Design review of the part built by this model. Coordinates are the model's own, in mm. Face numbers are marked on the shaded views. Coordinates: 2 decimals unless noted, no trailing zeros. Loops run counter-clockwise (first coordinate to the right, second up) from the corner with the lowest first, then second, coordinate; pieces in that order, holes last. Notation, with made-up numbers: M 25,-24.75 L 30,-24.75 A17 ccw 30,-3.75 Z; hole C 36.5,-34 d2. An arc over 180 degrees is marked long. One line per item, written item: value.
```python
from build123d import *

# Parameters (mm, degrees)
F0_W      = 67
F0_H      = 50
F1_DEPTH  = 70
F3_DEPTH  = 1.5
F4_W      = 29
F4_H      = 3.3
F5_DEPTH  = 67.001
F6_R      = 3.15
F7_DEPTH  = 9.2
F9_R      = 20
F10_DEPTH = 1.5
F12_R     = 20
F13_DEPTH = 1.5


with BuildPart() as f1:
    # F0 (on Top) → F1 (new body)
    with BuildSketch(Plane.XY):
        with Locations((33.5, 25)):
            Rectangle(F0_W, F0_H)
    extrude(amount=F1_DEPTH)

    # F2 (on face) → F3 (cut)
    with BuildSketch(Plane.XZ):
        Polygon((8.3138438763, 70), (0, 70), (0, 65.2), (28.9057142857, 35), (0, 4.8), (0, 0), (8.3138438763, 0), (33.5, 26.3138944576), (58.6861561237, 0), (67, 0), (67, 4.8), (38.0942857143, 35), (67, 65.2), (67, 70), (58.6861561237, 70), (33.5, 43.6861055424), align=None)
    extrude(amount=-F3_DEPTH, mode=Mode.SUBTRACT)

    # F4 (on face) → F5 (cut, through all)
    with BuildSketch(Plane.YZ.offset(67)):
        with BuildLine():
            Line((50, 36.5), (43.4544826719, 36.5))
            ThreePointArc((43.4544826719, 36.5), (8, 27), (43.4544826719, 17.5))
            Line((43.4544826719, 17.5), (50, 17.5))
            Line((50, 17.5), (50, 36.5))
        make_face()
        with Locations((35.5, 59.15)):
            Rectangle(F4_W, F4_H)
    extrude(amount=-F5_DEPTH, mode=Mode.SUBTRACT)

    # F6 (on face) → F7 (cut, through all)
    with BuildSketch(Plane.XY.offset(70)):
        with Locations((33.5, 41.7)):
            Circle(F6_R)
    extrude(amount=-F7_DEPTH, mode=Mode.SUBTRACT)

    # F9 (on offset) → F10 (cut)
    with BuildSketch(Plane.YZ.offset(54.5)):
        with Locations((27, 27)):
            Circle(F9_R)
    extrude(amount=F10_DEPTH, mode=Mode.SUBTRACT)

    # F12 (on offset) → F13 (cut)
    with BuildSketch(Plane(origin=(12.5, 0, 0), x_dir=(0, -1, 0), z_dir=(-1, 0, 0))):
        with Locations((-27, 27)):
            Circle(F12_R)
    extrude(amount=F13_DEPTH, mode=Mode.SUBTRACT)


solid = f1.part
```
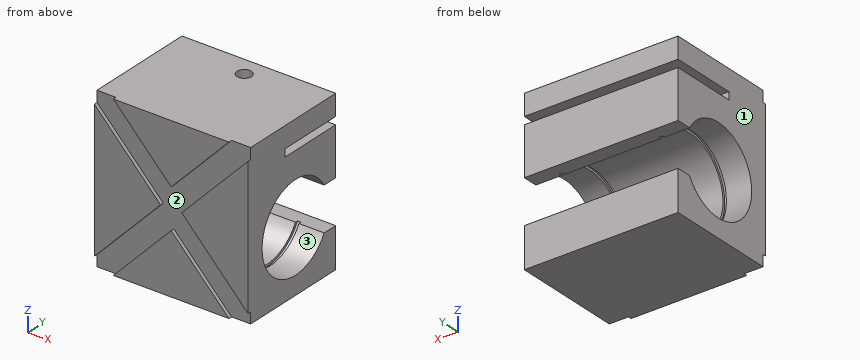
(1) To check wall thickness, follow line 1 along X through (y, z) = (9, 20.5); line 2 along Z through (x, y) = (61, 27); line 3 along Z through (x, y) = (55, 27). State the ranges of each line that lie inside material, in increasing order. Write a range as [from, to].
Reply:
line 1: x = [0, 11], [12.5, 54.5], [56, 67]
line 2: z = [0, 8], [46, 57.5], [60.8, 70]
line 3: z = [0, 7], [47, 57.5], [60.8, 70]
(2) Insertion check: pin 1 (4 mm diameter, centred on x = 33.5, y = 41.7, fed in from +Z); pin 2 (2.5 mm diameter, centred on x = 49.5, z = 59.5, fed in from +Y). Each pin has a flat end and moves straight along its axis. Give the tip position at first contact, or say it passes through.
Reply:
pin 1: stops at z = 57.5
pin 2: stops at y = 21
(3) We need section A-A on y = 27. State the section outline as (x, z) points.
Reply:
outline: M 0,0 L 67,0 L 67,8 L 56,8 L 56,7 L 54.5,7 L 54.5,8 L 12.5,8 L 12.5,7 L 11,7 L 11,8 L 0,8 Z; M 0,46 L 11,46 L 11,47 L 12.5,47 L 12.5,46 L 54.5,46 L 54.5,47 L 56,47 L 56,46 L 67,46 L 67,57.5 L 0,57.5 Z; M 0,60.8 L 67,60.8 L 67,70 L 0,70 Z
(4) We need section C-C on y = 16. State the section outline as (x, z) points, then the cut area to 3 significant figures.
Reply:
outline: M 0,0 L 67,0 L 67,11.51 L 56,11.51 L 56,10.3 L 54.5,10.3 L 54.5,11.51 L 12.5,11.51 L 12.5,10.3 L 11,10.3 L 11,11.51 L 0,11.51 Z; M 0,42.49 L 11,42.49 L 11,43.7 L 12.5,43.7 L 12.5,42.49 L 54.5,42.49 L 54.5,43.7 L 56,43.7 L 56,42.49 L 67,42.49 L 67,70 L 0,70 Z
area: 2,610 mm2
(5) We need section D-D on x = 57. State the section outline as (y, z) points.
Reply:
outline: M 0,0 L 50,0 L 50,17.5 L 43.45,17.5 A19 cw long 43.45,36.5 L 50,36.5 L 50,57.5 L 21,57.5 L 21,60.8 L 50,60.8 L 50,70 L 0,70 L 0,68.24 L 1.5,68.24 L 1.5,54.75 L 0,54.75 L 0,15.25 L 1.5,15.25 L 1.5,1.76 L 0,1.76 Z
(6) Mouldability with a two-part tool opening along X and no side actions: class the marked faces 1, 2 and 3 as released by +X, released by -X, zero draft, split by the parting line, or undercut.
Reply:
face 1: released by -X
face 2: undercut
face 3: zero draft
